Could you check a few things on this model? Use its own coordinates, in mm. A direction names the side the tool comes from. Coordinates: 2 decimals unless noted, no trailing zeros. Loops run counter-clockwise (first coordinate to the right, second up) from the corner with the lowest first, then second, coordinate; pieces in that order, holes last. Notation, with made-up numbers: (42, 19.25) - (92, 19.25) arc R24 cw to (92, 34.25) - close; hole circle Ø5 at (44.25, 78.25). An arc over 180 degrees is marked (long way). Use CSV: the item, a comma, the result in double quotes.
Autodesk Inventor part; units mm, degrees
ref_plane "YZ Plane" through (0, 0, 0) normal (1, 0, 0) x (0, 1, 0)
ref_plane "XY Plane" through (0, 0, 0) normal (0, 0, 1) x (1, 0, 0)
sketch "Sketch1" plane through (0, 0, 0) normal (0, 0, 1) x (1, 0, 0)
  circle A0 centre (0, 0) radius 57.5
  circle A1 centre (0, 0) radius 60.5
  dimension "d0" = 115
  dimension "d1" = 121
extrude "Extrusion1" add sketch "Sketch1" along normal blind 7
ref_plane "Work Plane1" through (0, -59, 0) normal (0, 1, 0) x (-1, 0, 0)
sketch "Sketch2" plane through (0, -59, 0) normal (0, 1, 0) x (-1, 0, 0)
  point P0 (0, 0)
sketch "Sketch3" plane through (0, -59, 0) normal (0, 1, 0) x (-1, 0, 0)
  line L0 (0, 0) -> (-70, 0)
  line L1 (-70, 0) -> (-70, 7)
  line L2 (-70, 7) -> (0, 7)
  line L3 (0, 7) -> (0, 0)
  line L4 (0, 0) -> (70, 0)
  line L5 (70, 0) -> (70, 7)
  line L6 (70, 7) -> (0, 7)
  dimension "d5" = 70
  dimension "d6" = 7
extrude "Extrusion2" add sketch "Sketch3" along normal mid plane 3
sketch "Sketch4" plane through (0, 0, 7) normal (0, 0, 1) x (1, 0, 0)
  line L0 (48, 5) -> (73, 5)
  line L1 (73, 5) -> (73, -5)
  line L2 (73, -5) -> (48, -5)
  line L3 (48, -5) -> (48, 5)
  line L4 (48, 5) -> (73, -5) construction
  line L5 (73, 5) -> (48, -5) construction
  line L6 (48, 1.5) -> (73, 1.5)
  line L7 (73, 1.5) -> (73, -1.5)
  line L8 (73, -1.5) -> (48, -1.5)
  line L9 (48, -1.5) -> (48, 1.5)
  line L10 (48, 1.5) -> (73, -1.5) construction
  line L11 (73, 1.5) -> (48, -1.5) construction
  line L12 (0, 0) -> (0, -12.7)
  line L13 (-48, 5) -> (-73, 5)
  line L14 (-73, 5) -> (-73, -5)
  line L15 (-73, -5) -> (-48, -5)
  line L16 (-48, -5) -> (-48, 5)
  line L17 (-48, 5) -> (-73, -5) construction
  line L18 (-73, 5) -> (-48, -5) construction
  line L19 (-48, 1.5) -> (-73, 1.5)
  line L20 (-73, 1.5) -> (-73, -1.5)
  line L21 (-73, -1.5) -> (-48, -1.5)
  line L22 (-48, -1.5) -> (-48, 1.5)
  line L23 (-48, 1.5) -> (-73, -1.5) construction
  line L24 (-73, 1.5) -> (-48, -1.5) construction
  line L25 (-70, -60.5) -> (70, -60.5)
  line L26 (36.5, -75) -> (-36.5, -75)
  line L27 (-36.5, -75) -> (-36.5, -46)
  line L28 (-36.5, -46) -> (36.5, -46)
  line L29 (36.5, -46) -> (36.5, -75)
  line L30 (36.5, -75) -> (-36.5, -46) construction
  line L31 (-36.5, -75) -> (36.5, -46) construction
  line L32 (36.5, -60.5) -> (-36.5, -60.5)
  arc A0 (60.293, -5) -> (60.293, 5) centre (0, 0) ccw
  arc A1 (-60.293, 5) -> (-60.293, -5) centre (0, 0) ccw
  arc A2 (-36.5, -48.2494) -> (36.5, -48.2494) centre (0, 0) ccw
  point P0 (60.5, 0)
  point P1 (60.5, 0)
  point P2 (-60.5, 0)
  point P3 (-60.5, 0)
  point P4 (0, -60.5)
  point P5 (-60.4814, -1.5)
  point P6 (-60.4814, 1.5)
  point P7 (0, -60.5)
  point P8 (60.4814, -1.5)
  point P9 (60.4814, 1.5)
  dimension "d10" = 25
  dimension "d11" = 10
  dimension "d12" = 25
  dimension "d13" = 3
  dimension "d17" = 73
  dimension "d18" = 29
extrude "Extrusion3" add sketch "Sketch4" against normal blind 7 contours L0 L1 L6 A0 | L8 L1 L2 A0 | A1 L19 L14 L13 | A1 L15 L14 L21 | L27 A2 L25 | A2 L29 L25
fillet "Fillet1" radius 8 5 edges at (-60.293, -5, 3.5) (-60.293, 5, 3.5) (60.293, -5, 3.5) (36.5, -57.5, 3.5) (-36.5, -57.5, 3.5)
properties part number "EXTRA_PARA CORTE DE TUBO"
(1) Suppose I cut it at B-B (x = -53.5). Write out the boundary of the cut face in (y, z), plus the area to 3 significant figures.
Computed:
outline,"(-60.5, 0) - (-57.5, 0) - (-57.5, 7) - (-60.5, 7) - close; (-28.25, 0) - (-21.07, 0) - (-21.07, 7) - (-28.25, 7) - close; (21.07, 0) - (28.25, 0) - (28.25, 7) - (21.07, 7) - close"
area,"121 mm²"
(2) Thinking about a two-plate mould opening in X: for faces 1 (the face through (-12.465, 56.133, 3.451)), 2 (the face through (62.1, -6.88, 3.45)), 3 (the face through (5, -58, 7)), which applies, +X half, -X half, draft (parallel to the pull), parting line (faces both ways), or undercut?
Computed:
face 1,"undercut"
face 2,"+X half"
face 3,"draft"
(3) Suppose I cut it at A-A (x = 6). Write out the boundary of the cut face in (y, z).
Computed:
outline,"(-60.5, 0) - (-57.19, 0) - (-57.19, 7) - (-60.5, 7) - close; (57.19, 0) - (60.2, 0) - (60.2, 7) - (57.19, 7) - close"
(4) Please list where these lines run through material, in increasing order: line 1 (Y direction, x = 0, z = 3); line 2 (Y direction, x = -66, z = 5.5); line 3 (Y direction, x = -49, z = 2).
Computed:
line 1,"y = -60.5 to -57.5, 57.5 to 60.5"
line 2,"y = -60.5 to -57.5, -5.1 to -1.5, 1.5 to 5.1"
line 3,"y = -60.5 to -57.5, -35.49 to -30.09, 30.09 to 35.49"
(5) Suppose I cut it at C-C (y = 50.5). Write out the boundary of the cut face in (x, z).
Computed:
outline,"(-33.32, 0) - (-27.5, 0) - (-27.5, 7) - (-33.32, 7) - close; (27.5, 0) - (33.32, 0) - (33.32, 7) - (27.5, 7) - close"
(6) Will these pins go through, and if not, where does the flat tip stop? pin 1 (2.5 mm diameter, centred on y = -59.5, z = 5, fed in from -X); pin 2 (1 mm diameter, centred on y = -49, z = 4, fed in from +X); pin 3 (2.5 mm diameter, centred on y = -58.5, z = 3.5, fed in from +X); pin 4 (1.7 mm diameter, centred on x = -70.5, z = 2.5, fed in from -Y).
Computed:
pin 1,"stops at x = -70"
pin 2,"stops at x = 36.5"
pin 3,"stops at x = 70"
pin 4,"stops at y = -60.5"
(7) Which directions (+Z, -Z, +X, -X, +Y, -Y) give clear straight access to the entire face, cutting with the end or side of a thin tool? Please do faces 4 (the face through (-70, 5, 4)), 5 (the face through (67, 5, 4)), 6 (the face through (-38.781, -55.094, 3.451)), 7 (the face through (67, 1.5, 4)), 8 (the face through (-1, -60.5, 4)).
Computed:
face 4,"+Z, -Z, -X, +Y"
face 5,"+Z, -Z, +X, +Y"
face 6,"+Z, -Z, -X"
face 7,"+Z, -Z, +X"
face 8,"+Z, -Z, +X, -X, -Y"
